Check sheet for the modelled part. Datum: model origin and axes. Units: mm. Give positions to 0.01 mm unless a question says otherwise; leave off trailing zeros. Loops run counter-clockwise (first coordinate to the right, second up) from the corner with the lowest first, then second, coordinate; pieces in that order, holes last. Notation, with made-up numbers: (43, 89) - (53, 89) arc R18 cw to (53, 101) - close; hole circle Ø5 at (-21.75, -12.5). An arc over 180 degrees is marked (long way). Use CSV: the item, a comma, the result in double quotes.
from build123d import *

# Parameters (mm, degrees)
SKETCH1_W           = 89
SKETCH1_H           = 99
BOSS_EXTRUDE1_DEPTH = 2
SKETCH2_R           = 1.6
CUT_EXTRUDE1_DEPTH  = 84.475926876
SKETCH3_R           = 1.6
CUT_EXTRUDE2_DEPTH  = 84.475926876


with BuildPart() as part:
    # Sketch1 → Boss-Extrude1 (new body)
    with BuildSketch(Plane.XY):
        with Locations((6.61978802, 16.462092452)):
            Rectangle(SKETCH1_W, SKETCH1_H)
    extrude(amount=BOSS_EXTRUDE1_DEPTH)

    # Sketch2 → Cut-Extrude1 (cut, through all)
    with BuildSketch(Plane.XY.offset(2)):
        with Locations((-31.88021198, 59.962092452)):
            Circle(SKETCH2_R)
        with Locations((45.11978802, 59.962092452)):
            Circle(SKETCH2_R)
        with Locations((-31.88021198, -27.037907548)):
            Circle(SKETCH2_R)
        with Locations((45.11978802, -27.037907548)):
            Circle(SKETCH2_R)
    extrude(amount=-CUT_EXTRUDE1_DEPTH, mode=Mode.SUBTRACT)

    # Sketch3 → Cut-Extrude2 (cut, through all)
    with BuildSketch(Plane.XY.offset(2)):
        with Locations((-15.88021198, 47.712092452)):
            Circle(SKETCH3_R)
        with Locations((-15.88021198, -20.787907548)):
            Circle(SKETCH3_R)
        with Locations((19.11978802, 62.712092452)):
            Circle(SKETCH3_R)
        with Locations((22.11978802, -18.787907548)):
            Circle(SKETCH3_R)
    extrude(amount=-CUT_EXTRUDE2_DEPTH, mode=Mode.SUBTRACT)


solid = part.part
1. Sectioned sample at A-A, the plane x = -31.5. Record the boundary of the cut face in (y, z).
Completed:
outline,"(-33.04, 0) - (-28.59, 0) - (-28.59, 2) - (-33.04, 2) - close; (-25.48, 0) - (58.41, 0) - (58.41, 2) - (-25.48, 2) - close; (61.52, 0) - (65.96, 0) - (65.96, 2) - (61.52, 2) - close"
2. Scan line: line 1 along X through (y, z) = (-18.5, 0.9). Record every from-to range of solid material in increasing order.
Completed:
line 1,"x = -37.88 to 20.55, 23.69 to 51.12"
3. Release check for a two-part mould opening along Y. For faces 1 (the face through (-31.142, 58.543, 1.014)), 2 (the face through (6, 17, 0)), 3 (the face through (6, -33.038, 1)), 4 (the face through (6, 65.962, 1)) record: released by +Y, released by -Y, zero draft, split by the parting line, or undercut.
Completed:
face 1,"undercut"
face 2,"zero draft"
face 3,"released by -Y"
face 4,"released by +Y"
